from build123d import *

# Parameters (mm, degrees)
SKETCH1_R           = 35
SKETCH1_R_2         = 34
BOSS_EXTRUDE1_DEPTH = 200
SKETCH2_R           = 34
SKETCH2_R_2         = 32.9
BOSS_EXTRUDE2_DEPTH = 2
BOSS_EXTRUDE3_START = 30
SKETCH3_R           = 33.9
SKETCH3_R_2         = 32.9
BOSS_EXTRUDE3_DEPTH = 30
SKETCH4_R           = 33.9
BOSS_EXTRUDE4_DEPTH = 2
SKETCH5_R           = 5
CUT_EXTRUDE1_DEPTH  = 2
SKETCH7_R           = 3
SKETCH7_R_2         = 2
BOSS_EXTRUDE8_DEPTH = 160
FILLET2_R           = 2
SKETCH8_R           = 2
CUT_EXTRUDE2_DEPTH  = 2
SKETCH9_R           = 4.5
SKETCH9_R_2         = 3.5
BOSS_EXTRUDE9_DEPTH = 150
FILLET3_R           = 2


with BuildPart() as part:
    # Sketch1 → Boss-Extrude1 (new body)
    with BuildSketch(Plane(origin=(0, 0, 0), x_dir=(1, 0, 0), z_dir=(0, 1, 0))):
        with Locations(Location((0, 0, 0), (0, 0, 270))):
            Circle(SKETCH1_R)
        with Locations(Location((0, 0, 0), (0, 0, 270))):
            Circle(SKETCH1_R_2, mode=Mode.SUBTRACT)
    extrude(amount=BOSS_EXTRUDE1_DEPTH)

    # Sketch2 → Boss-Extrude2 (add)
    with BuildSketch(Plane.XZ):
        with Locations(Location((0, 0, 0), (0, 0, 270))):
            Circle(SKETCH2_R)
        with Locations(Location((0, 0, 0), (0, 0, 270))):
            Circle(SKETCH2_R_2, mode=Mode.SUBTRACT)
    extrude(amount=-BOSS_EXTRUDE2_DEPTH)

    # Sketch3 → Boss-Extrude3 (add)
    with BuildSketch(Plane.XZ.offset(BOSS_EXTRUDE3_START)):
        with Locations(Location((0, 0, 0), (0, 0, 90))):
            Circle(SKETCH3_R)
        with Locations(Location((0, 0, 0), (0, 0, 270))):
            Circle(SKETCH3_R_2, mode=Mode.SUBTRACT)
    extrude(amount=-BOSS_EXTRUDE3_DEPTH)

    # Sketch4 → Boss-Extrude4 (add)
    with BuildSketch(Plane.XZ.offset(30)):
        with Locations(Location((0, 0, 0), (0, 0, 90))):
            Circle(SKETCH4_R)
    extrude(amount=-BOSS_EXTRUDE4_DEPTH)

    # Sketch5 → Cut-Extrude1 (cut)
    with BuildSketch(Plane.XZ.offset(30)):
        with Locations(Location((0, 0, 0), (0, 0, 270))):
            Circle(SKETCH5_R)
    extrude(amount=-CUT_EXTRUDE1_DEPTH, mode=Mode.SUBTRACT)

    # Sketch7 → Boss-Extrude8 (add)
    with BuildSketch(Plane(origin=(0, 2, 0), x_dir=(1, 0, 0), z_dir=(0, 1, 0))):
        with Locations((32, 0)):
            Circle(SKETCH7_R)
        with Locations(Location((32, 0, 0), (0, 0, 64.84439143))):
            Circle(SKETCH7_R_2, mode=Mode.SUBTRACT)
    extrude(amount=BOSS_EXTRUDE8_DEPTH)

    # Fillet2
    # the kernel refuses this fillet: 2 mm, written as the material it adds along each edge
    with BuildSketch(Plane(origin=(33.921875, 162, 2.303561695), x_dir=(-0.11187189352087389, 0, 0.9937226370773962), z_dir=(0, -1, 0))) as fillet2_piece_1:
        with BuildLine():
            CenterArc((2.923029325, 1.998037582), FILLET2_R, 178.057565486, 94.480798786)
            ThreePointArc((0.924178552, 2.06582835), (0.66436101, 0.942424954), (0, 0))
            ThreePointArc((0, 0), (1.505802985, -0.033361112), (3.011605971, 0))
        make_face()
    extrude(amount=160)
    with BuildSketch(Plane(origin=(33.921875, 162, -2.303561695), x_dir=(-0.11187189352087391, 0, -0.993722637077396), z_dir=(0, -1, 0))) as fillet2_piece_2:
        with BuildLine():
            CenterArc((2.923029325, -1.998037582), FILLET2_R, 87.461635728, 94.480798786)
            ThreePointArc((0.924178552, -2.06582835), (0.66436101, -0.942424954), (0, 0))
            ThreePointArc((0, 0), (1.505802985, 0.033361112), (3.011605971, 0))
        make_face()
    extrude(amount=160)

    # Sketch8 → Cut-Extrude2 (cut)
    with BuildSketch(Plane(origin=(0, -28, 0), x_dir=(1, 0, 0), z_dir=(0, 1, 0))):
        with Locations(Location((31.18904707, 0, 0), (0, 0, 270))):
            Circle(SKETCH8_R)
    extrude(amount=-CUT_EXTRUDE2_DEPTH, mode=Mode.SUBTRACT)

    # Sketch9 → Boss-Extrude9 (add)
    with BuildSketch(Plane(origin=(0, 200, 0), x_dir=(1, 0, 0), z_dir=(0, 1, 0))):
        with Locations((27.223611076, -27.223611076)):
            Circle(SKETCH9_R)
        with Locations(Location((27.223611076, -27.223611076, 0), (0, 0, 270))):
            Circle(SKETCH9_R_2, mode=Mode.SUBTRACT)
    extrude(amount=-BOSS_EXTRUDE9_DEPTH)

    # Fillet3
    fillet3_edges = [part.edges().sort_by_distance(p)[0] for p in [
        (26.580781197, 125, 22.769762207),
        (22.769762207, 125, 26.580781197),
    ]]
    fillet(fillet3_edges, radius=FILLET3_R)


solid = part.part
CAD build for the part. Positions are in the model's coordinates, mm. A direction names the side the tool comes from. Round coordinates to 2 decimals unless told otherwise and drop trailing zeros. Write each loop counter-clockwise with the first axis right and the second up, starting at its lowest first coordinate (ties: lowest second). Pieces come first, ordered by that corner, then holes. Notation, with made-up numbers: M 69.25,89 L 82.25,89 A33 ccw 82.25,118 Z; hole C 80,-29.5 d6. An arc over 180 degrees is marked long. Put each result on its own line as item: value. Start each with the question number.
1) Pull direction Y, two halves, no side cores. Call faces 1 (the flat face through (0, -30, 7)), 2 (the cylindrical face through (-4.88, -29.01, 1.08)), 3 (the flat face through (30, 2, 1)): pulls with the +Y half, pulls with the -Y half, needs draft (parallel to the pull), parting line crosses it, or undercut.
2) Saw through at B-B, the plane x = -12.5. Write the cut outline in (y, z), and give its area (3 significant figures).
3) Drill centre lines: probe 1 along X at (y, z) = (-29.6, 0); probe 2 along X at (y, z) = (-13.25, 0); probe 3 along Z at (x, y) = (0, 86). Where is each one in solid material? Low to high. Write a range as [from, to].
4) Pin check, flat tips, straight feed: pin 1 Ø3 at (y, z) = (105, 6.5) entering from -X; pin 2 Ø4 at (x, y) = (23.5, 60.5) entering from +Z; pin 3 Ø6 at (x, z) = (0, 0) entering from -Y; pin 4 Ø6 at (x, y) = (-4.5, 145.5) entering from -Z. Stop position of each tip, or through.
5) Saw through at C-C, the plane z = -13. Write the cut outline in (x, y).
6) 3-axis set-ups, long thin cutter, end or side, ignore diameter. For faces 4 (the cylindrical face through (30.694, 126.05, 26.768)), 5 (the cylindrical face through (29, 81, 0)), 6 (the cylindrical face through (-33.61, -15.21, -4.41)): which of +Z, -Z, +X, -X, +Y, -Y reach the whole face in a straight line?
7) Saw through at D-D, the plane y = 23. Write the cut outline in (x, z), and give its area (3 significant figures).
8) Saw through at A-A, the plane x = 0. Write the cut outline in (y, z).
Resolved:
1. face 1: pulls with the -Y half
1. face 2: needs draft
1. face 3: undercut
2. outline: M -30,-31.51 L 0,-31.51 L 0,-32.69 L 200,-32.69 L 200,-31.62 L 2,-31.62 L 2,-30.43 L -28,-30.43 L -28,30.43 L 2,30.43 L 2,31.62 L 200,31.62 L 200,32.69 L 0,32.69 L 0,31.51 L -30,31.51 Z
2. area: 620 mm²
3. probe 1: [-33.9, -5], [5, 29.19], [33.19, 33.9]
3. probe 2: [-33.9, -32.9], [32.9, 33.9]
3. probe 3: [-35, -34], [34, 35]
4. pin 1: x = -34.64
4. pin 2: z = 31.38
4. pin 3: through
4. pin 4: z = -34.97
5. outline: M -32.5,0 L -31.31,0 L -31.31,-30 L 31.31,-30 L 31.31,0 L 32.5,0 L 32.5,200 L 31.42,200 L 31.42,2 L 30.22,2 L 30.22,-28 L -30.22,-28 L -30.22,2 L -31.42,2 L -31.42,200 L -32.5,200 Z
6. face 4: +Y, -Y
6. face 5: +Y
6. face 6: -Y
7. outline: C 0,0 d70; hole C 32,0 d4; hole M 31.77,-2.99 A3 cw 31.77,2.99 A2 ccw 33.58,5.3 A34 ccw long 33.58,-5.3 A2 ccw Z
7. area: 232 mm²
8. outline: M -30,-33.9 L 0,-33.9 L 0,-35 L 200,-35 L 200,-34 L 2,-34 L 2,-32.9 L -28,-32.9 L -28,-5 L -30,-5 Z; M -30,5 L -28,5 L -28,32.9 L 2,32.9 L 2,34 L 200,34 L 200,35 L 0,35 L 0,33.9 L -30,33.9 Z
